Check sheet for the drawn part. Datum: minimum x, y, z corner. Units: mm. A direction names the side the tool comes from. Give positions to 0.01 mm unless a question says otherwise; leave off trailing zeros. Order: outer loops, then holes, each group sorted by start corner. A loop starts at its lowest first (then second) coordinate and runs counter-clockwise, first axis right, second up.
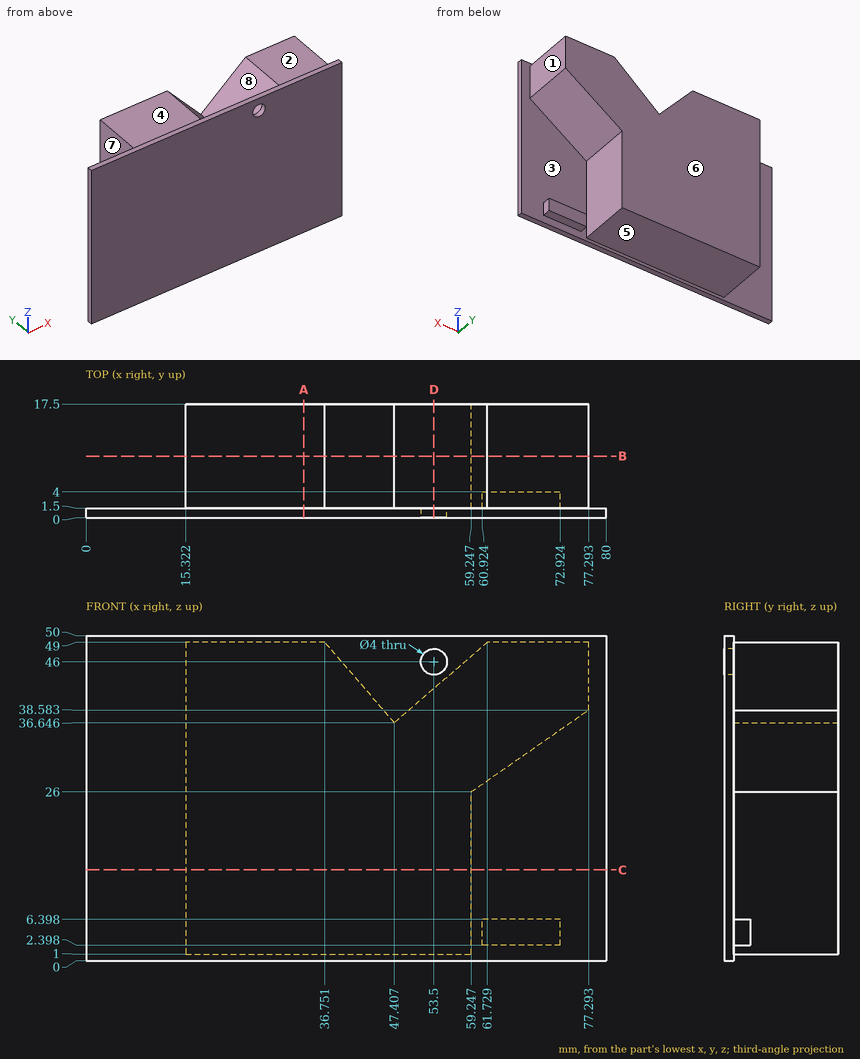
Item 1: Sectioned sample at C-C (z = 14). Enter the section's corners in (x, y).
Reported:
outline: (0, 0) - (80, 0) - (80, 1.5) - (59.25, 1.5) - (59.25, 17.5) - (15.32, 17.5) - (15.32, 1.5) - (0, 1.5) - close
Item 2: Draft check along Z on the marked faces 1, 2 and 3. Enter one of: released by +Z, released by -Z, zero draft, split by the parting line, or undercut.
Reported:
face 1: zero draft
face 2: released by +Z
face 3: undercut
Item 3: Sectioned sample at B-B (y = 9.5). Enter the section's corners in (x, z), and give its area (3 significant figures).
Reported:
outline: (15.32, 1) - (59.25, 1) - (59.25, 26) - (77.29, 38.58) - (77.29, 49) - (61.73, 49) - (47.41, 36.65) - (36.75, 49) - (15.32, 49) - close
area: 2,260 mm2
Item 4: Gauge pin test, flat ends, axial feed: pin 1 (8 mm diameter, centred on y = 8, z = 33.5, fed in from -X); pin 2 (8 mm diameter, centred on x = 38, y = 10.5, fed in from -Z); pin 3 (4 mm diameter, centred on x = 36.5, y = 15.5, fed in from +Z); pin 4 (3.5 mm diameter, centred on x = 53.5, z = 46, fed in from +Y). Record the tip position at first contact, or that the pin passes through.
Reported:
pin 1: stops at x = 15.32
pin 2: stops at z = 1
pin 3: stops at z = 49
pin 4: passes through
Item 5: Sectioned sample at D-D (x = 53.5). Enter the section's corners in (y, z).
Reported:
outline: (0, 0) - (1.5, 0) - (1.5, 1) - (17.5, 1) - (17.5, 41.9) - (1.5, 41.9) - (1.5, 44) - (0, 44) - close; (0, 48) - (1.5, 48) - (1.5, 50) - (0, 50) - close
Item 6: Sectioned sample at A-A (x = 33.5). Enter the section's corners in (y, z), and give its area (3 significant figures).
Reported:
outline: (0, 0) - (1.5, 0) - (1.5, 1) - (17.5, 1) - (17.5, 49) - (1.5, 49) - (1.5, 50) - (0, 50) - close
area: 843 mm2
Item 7: Set-up check for the marked faces 4, 5, 6, 7 and 8: record each of +Z, -Z, +X, -X, +Y, -Y from which the full face is reachable in a straight line by a thin tool's end or side.
Reported:
face 4: +Z, +X, -X, +Y
face 5: -Z, +X, -X, +Y
face 6: +Z, -Z, +X, -X, +Y
face 7: +Z, -Z, -X, +Y
face 8: +Z, +Y
Item 8: Scan lines: L1, parallel to X at y = 0.8, z = 46; L2, parallel to Z at x = 53.5, y = 0.9; L3, parallel to Y at x = 56, z = 45. Record each from-to range of solid material in increasing order.
Reported:
L1: x = 0 to 51.5, 55.5 to 80
L2: z = 0 to 44, 48 to 50
L3: y = 0 to 1.5
